```python
from build123d import *

# Parameters (mm, degrees)
SKETCH1_W           = 226
SKETCH1_H           = 146
SKETCH1_W_2         = 220
SKETCH1_H_2         = 140
BOSS_EXTRUDE1_DEPTH = 150
SKETCH1_4_W         = 220
SKETCH1_4_H         = 140
BOSS_EXTRUDE2_DEPTH = 3
SKETCH2_W           = 266
SKETCH2_H           = 186
SKETCH2_W_2         = 220
SKETCH2_H_2         = 140
BOSS_EXTRUDE3_DEPTH = 3
FILLET1_R           = 10
SKETCH3_R           = 4
CUT_EXTRUDE1_DEPTH  = 221.993212565


with BuildPart() as part:
    # Sketch1 → Boss-Extrude1 (new body)
    with BuildSketch(Plane(origin=(0, 0, 0), x_dir=(1, 0, 0), z_dir=(0, 1, 0))):
        Rectangle(SKETCH1_W, SKETCH1_H)
        Rectangle(SKETCH1_W_2, SKETCH1_H_2, mode=Mode.SUBTRACT)
    extrude(amount=BOSS_EXTRUDE1_DEPTH)

    # Sketch1_4 → Boss-Extrude2 (add)
    with BuildSketch(Plane(origin=(0, 0, 0), x_dir=(1, 0, 0), z_dir=(0, 1, 0))):
        Rectangle(SKETCH1_4_W, SKETCH1_4_H)
    extrude(amount=BOSS_EXTRUDE2_DEPTH)

    # Sketch2 → Boss-Extrude3 (add)
    with BuildSketch(Plane(origin=(0, 150, 0), x_dir=(1, 0, 0), z_dir=(0, 1, 0))):
        Rectangle(SKETCH2_W, SKETCH2_H)
        Rectangle(SKETCH2_W_2, SKETCH2_H_2, mode=Mode.SUBTRACT)
    extrude(amount=-BOSS_EXTRUDE3_DEPTH)

    # Fillet1
    fillet1_edges = [part.edges().sort_by_distance(p)[0] for p in [
        (-133, 148.5, 93),
        (-133, 148.5, -93),
        (133, 148.5, -93),
        (133, 148.5, 93),
    ]]
    fillet(fillet1_edges, radius=FILLET1_R)

    # Sketch3 → Cut-Extrude1 (cut, through all)
    with BuildSketch(Plane(origin=(0, 150, 0), x_dir=(1, 0, 0), z_dir=(0, 1, 0))):
        with Locations(Location((-122.5, -15, 0), (0, 0, 270))):
            Circle(SKETCH3_R)
        with Locations(Location((-122.5, -41.25, 0), (0, 0, 270))):
            Circle(SKETCH3_R)
        with Locations(Location((-122.5, -67.5, 0), (0, 0, 270))):
            Circle(SKETCH3_R)
        with Locations(Location((-107.5, -82.5, 0), (0, 0, 270))):
            Circle(SKETCH3_R)
        with Locations(Location((-77.5, -82.5, 0), (0, 0, 270))):
            Circle(SKETCH3_R)
        with Locations(Location((-45, -82.5, 0), (0, 0, 270))):
            Circle(SKETCH3_R)
        with Locations(Location((-15, -82.5, 0), (0, 0, 270))):
            Circle(SKETCH3_R)
        with Locations(Location((-45, 82.5, 0), (0, 0, 270))):
            Circle(SKETCH3_R)
        with Locations(Location((-15, 82.5, 0), (0, 0, 270))):
            Circle(SKETCH3_R)
        with Locations(Location((-77.5, 82.5, 0), (0, 0, 270))):
            Circle(SKETCH3_R)
        with Locations(Location((-107.5, 82.5, 0), (0, 0, 270))):
            Circle(SKETCH3_R)
        with Locations(Location((-122.5, 67.5, 0), (0, 0, 270))):
            Circle(SKETCH3_R)
        with Locations(Location((-122.5, 41.25, 0), (0, 0, 270))):
            Circle(SKETCH3_R)
        with Locations(Location((-122.5, 15, 0), (0, 0, 270))):
            Circle(SKETCH3_R)
        with Locations(Location((15, -82.5, 0), (0, 0, 270))):
            Circle(SKETCH3_R)
        with Locations(Location((45, -82.5, 0), (0, 0, 270))):
            Circle(SKETCH3_R)
        with Locations(Location((107.5, -82.5, 0), (0, 0, 270))):
            Circle(SKETCH3_R)
        with Locations(Location((122.5, -67.5, 0), (0, 0, 270))):
            Circle(SKETCH3_R)
        with Locations(Location((122.5, -41.25, 0), (0, 0, 270))):
            Circle(SKETCH3_R)
        with Locations(Location((122.5, -15, 0), (0, 0, 270))):
            Circle(SKETCH3_R)
        with Locations(Location((122.5, 15, 0), (0, 0, 270))):
            Circle(SKETCH3_R)
        with Locations(Location((122.5, 41.25, 0), (0, 0, 270))):
            Circle(SKETCH3_R)
        with Locations(Location((122.5, 67.5, 0), (0, 0, 270))):
            Circle(SKETCH3_R)
        with Locations(Location((107.5, 82.5, 0), (0, 0, 270))):
            Circle(SKETCH3_R)
        with Locations(Location((77.5, 82.5, 0), (0, 0, 270))):
            Circle(SKETCH3_R)
        with Locations(Location((45, 82.5, 0), (0, 0, 270))):
            Circle(SKETCH3_R)
        with Locations(Location((15, 82.5, 0), (0, 0, 270))):
            Circle(SKETCH3_R)
        with Locations(Location((77.5, -82.5, 0), (0, 0, 270))):
            Circle(SKETCH3_R)
    extrude(amount=-CUT_EXTRUDE1_DEPTH, mode=Mode.SUBTRACT)


solid = part.part
```
Input: part model. Units: mm. Frame: model coordinates. A direction names the side the tool comes from. Give positions to 0.01 mm unless a question says otherwise; leave off trailing zeros. Order: outer loops, then holes, each group sorted by start corner. A loop starts at its lowest first (then second) coordinate and runs counter-clockwise, first axis right, second up. Notation, with made-up numbers: (-24.75, 76.5) - (19.25, 76.5) arc R30 cw to (19.25, 111.5) - close; hole circle Ø2 at (20.5, -29.75). An arc over 180 degrees is marked (long way). Use a Markdown table: item, result.
(1) Section query D-D (z = -22.5). Output: boundary loops of the cut face in (x, y), then the cut area to 3 significant figures.
Computed values:
| item | result |
|---|---|
| outline | (-133, 147) - (-113, 147) - (-113, 0) - (113, 0) - (113, 147) - (133, 147) - (133, 150) - (110, 150) - (110, 3) - (-110, 3) - (-110, 150) - (-133, 150) - close |
| area | 1,680 mm2 |
(2) Section query C-C (x = -84.5). Output: boundary loops of the cut face in (y, z).
Computed values:
| item | result |
|---|---|
| outline | (0, -73) - (147, -73) - (147, -93) - (150, -93) - (150, -70) - (3, -70) - (3, 70) - (150, 70) - (150, 93) - (147, 93) - (147, 73) - (0, 73) - close |
(3) Section query B-B (y = 88.5). Output: boundary loops of the cut face in (x, z), then the cut area to 3 significant figures.
Computed values:
| item | result |
|---|---|
| outline | (-113, -73) - (113, -73) - (113, 73) - (-113, 73) - close; hole (-110, -70) - (110, -70) - (110, 70) - (-110, 70) - close |
| area | 2,200 mm2 |
(4) Section query A-A (z = 15). Output: boundary loops of the cut face in (x, y), then the cut area to 3 significant figures.
Computed values:
| item | result |
|---|---|
| outline | (-133, 147) - (-126.5, 147) - (-126.5, 150) - (-133, 150) - close; (-118.5, 147) - (-113, 147) - (-113, 0) - (113, 0) - (113, 147) - (118.5, 147) - (118.5, 150) - (110, 150) - (110, 3) - (-110, 3) - (-110, 150) - (-118.5, 150) - close; (126.5, 147) - (133, 147) - (133, 150) - (126.5, 150) - close |
| area | 1,630 mm2 |
(5) Line query: line 1 (Z direction, x = 53, y = 126.5); line 2 (X direction, y = 114, z = -58); line 3 (Y direction, x = -63.5, z = -14). Output: solid intervals per line, ascending. Write a range as from..to.
Computed values:
| item | result |
|---|---|
| line 1 | z = -73..-70, 70..73 |
| line 2 | x = -113..-110, 110..113 |
| line 3 | y = 0..3 |
(6) Access query for faces 4 (the cylindrical face through (-12.3, 148.52, -85.45)), 5 (the flat face through (-2, 72, 73)). Directions: +Z, -Z, +X, -X, +Y, -Y. A direction counts if a zero-diameter tool reaches every point of the face in a straight line with its end or side. Return the directions, or none.
Computed values:
| item | result |
|---|---|
| face 4 | +Y, -Y |
| face 5 | +Z, +X, -X, -Y |
(7) Pin query (flat end, axial travel): pin 1 (3 mm diameter, centred on x = -94, y = 117, fed in from +Z); pin 2 (10.5 mm diameter, centred on x = -15, z = -82.5, fed in from -Y); pin 3 (4 mm diameter, centred on x = -83.5, y = 126, fed in from -Z). Return the tip coordinate at first contact, or that it passes through.
Computed values:
| item | result |
|---|---|
| pin 1 | stops at z = 73 |
| pin 2 | stops at y = 147 |
| pin 3 | stops at z = -73 |
(8) Draft query along X for faces 1 (the flat face through (-2, 147, 81)), 2 (the flat face through (-2, 75, -70)), 3 (the cylindrical face through (-130.15, 148.48, 89.99)). Return one class per face: released by +X, released by -X, zero draft, split by the parting line, or undercut.
Computed values:
| item | result |
|---|---|
| face 1 | zero draft |
| face 2 | undercut |
| face 3 | released by -X |
